from build123d import *

# Parameters (mm, degrees)
F1_DEPTH = 2
F2_W     = 5
F2_H     = 5
F3_DEPTH = 0.5
F4_D     = 5


# Not quite as in the source:
# - a feature names something its author has since deleted; it is built from what else it names


with BuildPart() as f1:
    # F0 (on Top) → F1 (new body)
    with BuildSketch(Plane.XY):
        with BuildLine():
            ThreePointArc((-3.7594057481, 24.7157210783), (0, 25), (3.7594057481, 24.7157210783))
            ThreePointArc((3.7594057481, 24.7157210783), (4.209761495, 25.7828537011), (4.3634907466, 26.9308779389))
            ThreePointArc((4.3634907466, 26.9308779389), (-1.1480242378, 31.1406394339), (-3.7594057481, 24.7157210783))
        make_face()
        with BuildLine():
            ThreePointArc((-3.7594057481, 24.7157210783), (0, 22.5673871923), (3.7594057481, 24.7157210783))
            ThreePointArc((3.7594057481, 24.7157210783), (0, 25), (-3.7594057481, 24.7157210783))
        make_face()
        with BuildLine():
            ThreePointArc((-3.7594057481, 24.7157210783), (-16.2943986741, -18.9602893399), (25, 0))
            ThreePointArc((25, 0), (18.9602893399, 16.2943986741), (3.7594057481, 24.7157210783))
            ThreePointArc((3.7594057481, 24.7157210783), (0, 22.5673871923), (-3.7594057481, 24.7157210783))
        make_face()
    extrude(amount=F1_DEPTH)

    # F2 (on face) → F3 (join)
    with BuildSketch(Plane.XY.offset(2)):
        Polygon((-2.640592387, 25.1115851104), (-2.640592387, 2.5), (2.359407613, 2.5), (2.359407613, 25.1115851104), (-0.140592387, 25.1115851104), align=None)
        with BuildLine():
            Line((-2.640592387, 2.5), (-24.8746859277, 2.5))
            ThreePointArc((-24.8746859277, 2.5), (-24.9686518278, 1.2515693765), (-25, 0))
            ThreePointArc((-25, 0), (-24.9686518278, -1.2515693765), (-24.8746859277, -2.5))
            Line((-24.8746859277, -2.5), (-2.640592387, -2.5))
            Line((-2.640592387, -2.5), (-2.640592387, 2.5))
        make_face()
        with Locations((-0.140592387, 0)):
            Rectangle(F2_W, F2_H)
        with BuildLine():
            Line((24.8746859277, 2.5), (2.359407613, 2.5))
            Line((2.359407613, 2.5), (2.359407613, -2.5))
            Line((2.359407613, -2.5), (24.8746859277, -2.5))
            ThreePointArc((24.8746859277, -2.5), (24.9686518278, -1.2515693765), (25, 0))
            ThreePointArc((25, 0), (24.9686518278, 1.2515693765), (24.8746859277, 2.5))
        make_face()
        with BuildLine():
            Line((2.359407613, -2.5), (-2.640592387, -2.5))
            Line((-2.640592387, -2.5), (-2.640592387, -24.8601543005))
            ThreePointArc((-2.640592387, -24.8601543005), (-2.5000399327, -24.8746819142), (-2.359407613, -24.8884148896))
            Line((-2.359407613, -24.8884148896), (-0.140592387, -24.8884148896))
            Line((-0.140592387, -24.8884148896), (2.359407613, -24.8884148896))
            Line((2.359407613, -24.8884148896), (2.359407613, -2.5))
        make_face()
    extrude(amount=F3_DEPTH)

    # F4 (through all)
    with Locations(Plane(origin=(0, 0, 0), x_dir=(1, 0, 0), z_dir=(0, 0, -1))):
        with Locations((0, -26.9308779389)):
            Hole(F4_D / 2)


solid = f1.part
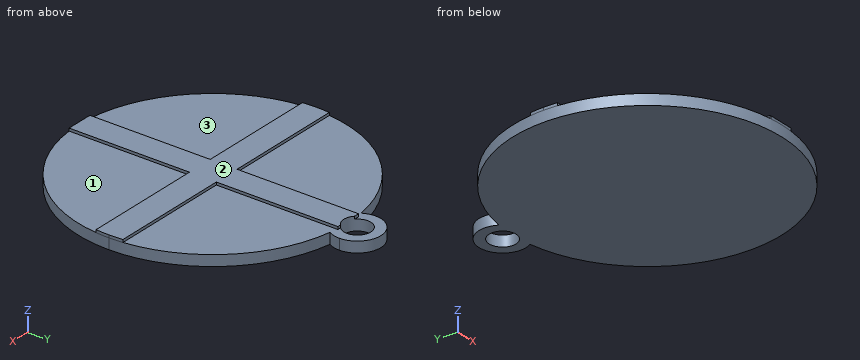
Geometry: final body of the model. Coordinates: model frame, mm. Face numbers are marked on the shaded views. A direction names the side the tool comes from. Coordinates: 2 decimals unless noted, no trailing zeros. Order: outer loops, then holes, each group sorted by start corner. A loop starts at its lowest first (then second) coordinate and runs counter-clockwise, first axis right, second up.
(1) Section query B-B (x = 15). Return the cut outline in (y, z), plus the area to 3 significant figures.
(2) Section query C-C (z = 1.5). Return the cut outline in (x, y).
(3) Material intervals for probe 1 along Y at (x, z) = (0, 1.7); probe 2 along Z at (x, y) = (4, -18); probe 3 along X at (y, z) = (3.5, 2.45), sorted ascending.
(4) Access query for the marked faces 1, 2 and 3. Directions: +Z, -Z, +X, -X, +Y, -Y. A direction counts if a zero-diameter tool reaches every point of the face in a straight line with its end or side. Return the directions, or none.
(5) Section query A-A (x = 0). Return the cut outline in (y, z), plus the area to 3 significant figures.
(6) First-contact query: pin 1 (0.6 mm diameter, centred on x = 14, z = 2.5, fed in from +Y); pin 2 (0.6 mm diameter, centred on x = -2, z = 2, fed in from +Y); pin 3 (8.5 mm diameter, centred on x = -10.5, y = 14, fed in from +Z); pin 4 (6 mm diameter, centred on x = 0, y = 26.93, fed in from +Z). Flat tips, straight axial feed; report the tip coordinate or a pass-through.
(7) Section query D-D (y = -20.5). Return the cut outline in (x, z).
Solution:
1. outline: (-20, 0) - (20, 0) - (20, 2) - (2.5, 2) - (2.5, 2.5) - (-2.5, 2.5) - (-2.5, 2) - (-20, 2) - close
1. area: 82.5 mm2
2. outline: (-3.76, 24.72) arc R25 ccw (long way) to (3.76, 24.72) arc R4.36 ccw (long way) to start; hole circle Ø5 at (0, 26.93)
3. probe 1: y = -25 to 24.43, 29.43 to 31.29
3. probe 2: z = 0 to 2
3. probe 3: x = -2.64 to 2.36
4. face 1: +Z, +X, -Y
4. face 2: +Z, +X, -X, +Y, -Y
4. face 3: +Z, -X, -Y
5. outline: (-25, 0) - (24.43, 0) - (24.43, 2.5) - (-24.89, 2.5) - (-24.89, 2) - (-25, 2) - close; (29.43, 0) - (31.29, 0) - (31.29, 2) - (29.43, 2) - close
5. area: 127 mm2
6. pin 1: stops at y = 2.5
6. pin 2: stops at y = 30.95
6. pin 3: stops at z = 2
6. pin 4: stops at z = 2.5
7. outline: (-14.31, 0) - (14.31, 0) - (14.31, 2) - (2.36, 2) - (2.36, 2.5) - (-2.64, 2.5) - (-2.64, 2) - (-14.31, 2) - close
